```python
from build123d import *


with BuildPart() as part:
    # Sketch1 → Elemento_elastico_en_serie (revolve)
    with BuildSketch(Plane.XY, mode=Mode.PRIVATE) as elemento_elastico_en_serie_sk:
        Polygon((0, 0), (1.82, 0), (3.8, -0.5), (2.6, -1.5), (3.8, -2.5), (2.6, -3.5), (3.8, -4.5), (2.6, -5.5), (3.8, -6.5), (2.6, -7.5), (3.8, -8.5), (2.6, -9.5), (3.8, -10.5), (2.6, -11.5), (3.8, -12.5), (2.6, -13.5), (3.8, -14.5), (2.6, -15.5), (3.8, -16.5), (2.6, -17.5), (1.82, -18), (0, -18), align=None)
    revolve(elemento_elastico_en_serie_sk.sketch.rotate(Axis((0, -22, 0), (0, 1, 0)), 90), axis=Axis((0, -22, 0), (0, 1, 0)))


solid = part.part
```
Input: part model. Units: mm. Frame: model coordinates. Give positions to 0.01 mm unless a question says otherwise; leave off trailing zeros. Order: outer loops, then holes, each group sorted by start corner. A loop starts at its lowest first (then second) coordinate and runs counter-clockwise, first axis right, second up. Notation, with made-up numbers: M -5,-14.75 L 5,-14.75 A34 cw 5,18.25 Z; hole C 40,-2 d8. An arc over 180 degrees is marked long. Return JSON: item names as keys, results as strings.
Item 1: Cut plane A-A (z = 3.25). State how many separate pieces and enclosed holes the cut face has, then the cut area to 3 significant figures.
Solutions:
{"separate pieces": "9", "enclosed holes": "0", "area": "20.5 mm^2"}
Item 2: Ray query, probe 1 along Z at (x, y) = (1.5, -3); probe 2 along Z at (x, y) = (1.75, -17); probe 3 along X at (y, z) = (-4.25, -1). Return the intervals inside material, ascending.
Solutions:
{"probe 1": "-2.83 to 2.83", "probe 2": "-2.68 to 2.68", "probe 3": "-3.35 to 3.35"}
Item 3: First-contact query: P1, Ø3, axis at x = -2, z = 2, coming from the -Y side; P2, Ø2, axis at x = 3, y = -3.5, coming from the +Z side. Flat tips, straight axial feed; report the tip coordinate or a pass-through.
Solutions:
{"P1": "y = -18", "P2": "z = 2.64"}
Item 4: Cut plane B-B (y = -9). Return loops of the section in (x, z).
Solutions:
{"outline": "C 0,0 d6.4"}
Item 5: Pull-direction query (Y, two-part tool) for faces 1 (the flat face through (0, -18, 0)), 2 (the conical face through (-0.8, -13.6, -2.6)); classes: +Y half, -Y half, draft (parallel to the pull), parting line (faces both ways), or undercut.
Solutions:
{"face 1": "-Y half", "face 2": "undercut"}
